Geometry: final body of the model. Coordinates: model frame, mm. Face numbers are marked on the shaded views. A direction names the side the tool comes from. Give positions to 0.01 mm unless a question says otherwise; leave off trailing zeros. Order: outer loops, then holes, each group sorted by start corner. A loop starts at its lowest first (then second) coordinate and runs counter-clockwise, first axis right, second up. Notation, with made-up numbers: (20.5, 54.25) - (66.5, 54.25) arc R9 ccw to (66.5, 61.25) - close; hole circle Ø3 at (-17, 38.25). An arc over 180 degrees is marked (long way). Write item = value, one per line. Start each with the question number.
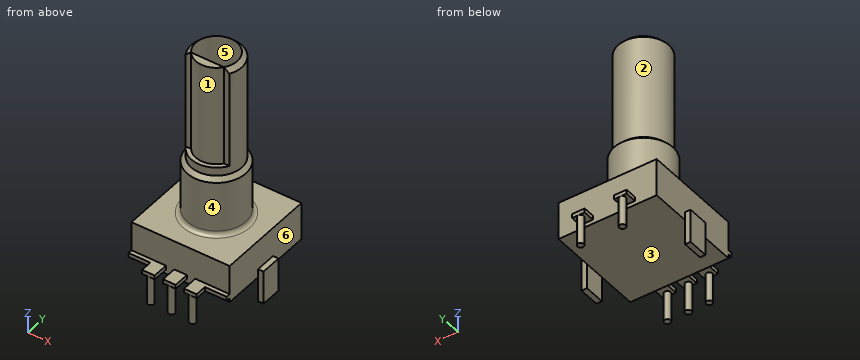
Autodesk Fusion 360 part; units mm, degrees
sketch "Skizze1" plane through (0, 0, 0) normal (0, 0, 1) x (1, 0, 0)
  line L0 (0, 0) -> (-11.7, 0)
  line L1 (-11.7, 0) -> (-11.7, 12)
  line L2 (-11.7, 12) -> (0, 12)
  line L3 (0, 12) -> (0, 0)
  dimension "d1" = 11.7
  dimension "d2" = 12
extrude "Extrusion1" add sketch "Skizze1" along normal blind 4.5
ref_plane "Arbeitsebene1" through (0, 0, 0.5) normal (0, 0, 1) x (1, 0, 0)
sketch "Skizze2" plane through (0, 0, 0.5) normal (0, 0, 1) x (1, 0, 0)
  line L0 (0, 12) -> (-11.7, 12)
  line L1 (-11.7, 12) -> (-11.7, 0)
  line L2 (-11.7, 0) -> (0, 0)
  line L3 (0, 0) -> (0, 12)
  line L4 (-8.35, 12) -> (-8.35, 19) construction
  line L5 (-3.35, 12) -> (-3.35, 19) construction
  line L6 (-8.35, 0) -> (-8.35, -5) construction
  line L7 (-5.85, 0) -> (-5.85, -5) construction
  line L8 (-3.35, 0) -> (-3.35, -5) construction
  line L9 (-7.6, 12) -> (-9.1, 12)
  line L10 (-9.1, 12) -> (-9.1, 13.375)
  line L11 (-9.1, 13.375) -> (-7.6, 13.375)
  line L12 (-7.6, 13.375) -> (-7.6, 12)
  line L13 (-2.6, 12) -> (-4.1, 12)
  line L14 (-4.1, 12) -> (-4.1, 13.375)
  line L15 (-4.1, 13.375) -> (-2.6, 13.375)
  line L16 (-2.6, 13.375) -> (-2.6, 12)
  line L17 (-2.6, 0) -> (-4.1, 0)
  line L18 (-4.1, 0) -> (-4.1, -1.875)
  line L19 (-4.1, -1.875) -> (-2.6, -1.875)
  line L20 (-2.6, -1.875) -> (-2.6, 0)
  line L21 (-6.6, 0) -> (-5.1, 0)
  line L22 (-5.1, 0) -> (-5.1, -1.875)
  line L23 (-5.1, -1.875) -> (-6.6, -1.875)
  line L24 (-6.6, -1.875) -> (-6.6, 0)
  line L25 (-9.1, 0) -> (-7.6, 0)
  line L26 (-7.6, 0) -> (-7.6, -1.875)
  line L27 (-7.6, -1.875) -> (-9.1, -1.875)
  line L28 (-9.1, -1.875) -> (-9.1, 0)
  line L29 (-9.1, 0) -> (-11.7, 0)
  line L30 (-11.7, 0) -> (-11.7, -0.5)
  line L31 (-11.7, -0.5) -> (-9.1, -0.5)
  line L32 (-9.1, -0.5) -> (-9.1, 0)
  line L33 (-2.6, 0) -> (0, 0)
  line L34 (0, 0) -> (0, -0.5)
  line L35 (0, -0.5) -> (-2.6, -0.5)
  line L36 (-2.6, -0.5) -> (-2.6, 0)
  circle A0 centre (-8.35, 13) radius 0.375
  circle A1 centre (-3.35, 13) radius 0.375
  circle A2 centre (-8.35, -1.5) radius 0.375
  circle A3 centre (-5.85, -1.5) radius 0.375
  circle A4 centre (-3.35, -1.5) radius 0.375
  line L37 (-11.7, 6) -> (0, 6) construction
  line L38 (-11.7, 7.25) -> (-12.35, 7.25)
  line L39 (-12.35, 7.25) -> (-12.35, 4.75)
  line L40 (-12.35, 4.75) -> (-11.7, 4.75)
  line L41 (-11.7, 4.75) -> (-11.7, 7.25)
  line L42 (0, 7.25) -> (0.65, 7.25)
  line L43 (0.65, 7.25) -> (0.65, 4.75)
  line L44 (0.65, 4.75) -> (0, 4.75)
  line L45 (0, 4.75) -> (0, 7.25)
  line L46 (-11.6, 7.25) -> (-11.6, 4.75)
  line L47 (-0.1, 7.25) -> (-0.1, 4.75)
  dimension "d7" = 5
  dimension "d8" = 5
  dimension "d9" = 1.5
  dimension "d11" = 0.5
  dimension "d12" = 0.75
  dimension "d13" = 0.75
  dimension "d14" = 0.75
  dimension "d15" = 0.75
  dimension "d16" = 0.75
  dimension "d17" = 7
  dimension "d18" = 7
  dimension "d19" = 7.5
  dimension "d20" = 7.5
  dimension "d21" = 7.5
  dimension "d26" = 0.75
  dimension "d27" = 0.75
  dimension "d28" = 13
  dimension "d46" = 2.5
extrude "Extrusion2" add sketch "Skizze2" along normal blind 0.5 contours A1 | L0 L13 L14 L15 L16 | L3 L42 L43 L44 L45 | A0 | L0 L9 L10 L11 L12 | L2 L20 L33 L34 L35 L36 | A4 | L2 L17 L18 L19 L20 L36 | L1 L38 L39 L40 L41 | A3 | L2 L21 L22 L23 L24 | L2 L28 L29 L30 L31 L32 | A2 | L2 L25 L26 L27 L28 L32
extrude "Extrusion3" add sketch "Skizze2" against normal blind 3.5 contours A1 | L3 L42 L43 L44 L45 | A0 | A4 | L1 L38 L39 L40 L41 | A3 | A2
ref_plane "Arbeitsebene2" through (0, 6, 0) normal (0, 1, 0) x (0, 0, 1)
sketch "Skizze3" plane through (0, 6, 0) normal (0, 1, 0) x (1, 0, 0)
  line L0 (-4.1, -1) -> (0, -1)
  line L1 (0, -1) -> (0, -4.5)
  line L2 (0, -4.5) -> (-11.7, -4.5)
  line L3 (-11.7, -4.5) -> (-11.7, -1)
  line L4 (-11.7, -1) -> (-7.6, -1)
  line L5 (-7.6, -1) -> (-7.6, -0.5)
  line L6 (-7.6, -0.5) -> (-11.7, -0.5)
  line L7 (-11.7, -0.5) -> (-11.7, 0)
  line L8 (-11.7, 0) -> (0, 0)
  line L9 (0, 0) -> (0, -0.5)
  line L10 (0, -0.5) -> (-4.1, -0.5)
  line L11 (-4.1, -0.5) -> (-4.1, -1)
  line L12 (-5.1, -1) -> (-5.1, -0.5)
  line L13 (-5.1, -0.5) -> (-6.6, -0.5)
  line L14 (-6.6, -0.5) -> (-6.6, -1)
  line L15 (-6.6, -1) -> (-5.1, -1)
  line L16 (-5.85, -4.5) -> (-5.85, -18.5)
  line L17 (-5.85, -4.5) -> (-1.85, -4.5)
  line L18 (-2.35, -5) -> (-2.35, -11)
  arc A0 (-1.85, -4.5) -> (-2.35, -5) centre (-1.85, -5) ccw
  line L19 (-2.35, -11) -> (-2.85, -11.5)
  line L20 (-2.85, -11.5) -> (-2.85, -23.9697)
  line L21 (-2.85, -23.9697) -> (-3.3803, -24.5)
  line L22 (-3.3803, -24.5) -> (-5.85, -24.5)
  line L23 (-5.85, -24.5) -> (-5.85, -4.5)
  dimension "d31" = 1
  dimension "d32" = 7
  dimension "d33" = 6
  dimension "d34" = 135
  dimension "d35" = 135
  dimension "d36" = 7
  dimension "d40" = 0.75
  dimension "d41" = 20
revolve "Drehen1" add sketch "Skizze3" angle 360 about axis through (-5.85, 6, 4.5) along (0, 0, 1) contours L2 L16 L17 L18 A0 L19 L20 L21 L22 L23
sketch "Skizze4" plane through (0, 0, 24.5) normal (0, 0, 1) x (-1, 0, 0)
  circle A0 centre (5.85, -6) radius 2.4697
  circle A1 centre (5.85, -6) radius 3
  line L0 (8.4481, -4.5) -> (3.2519, -4.5)
  arc A2 (8.4481, -4.5) -> (3.2519, -4.5) centre (5.85, -6) ccw
  line L1 (5.85, -4.5) -> (5.85, -9) construction
  dimension "d43" = 4.5
extrude "Extrusion4" cut sketch "Skizze4" against normal blind 12 contours A0 L0 | A0 A1 L0 A2 picked at (5.4755, -5.7331)
equation "d13 = d12"
equation "d14 = d12"
equation "d15 = d12"
equation "d16 = d12"
Q1. Section D-D, the plane y = 11. Return the cut outline in (x, z).
Q2. Material intervals for line 1 along Y through (x, z) = (-5.85, 20.5); line 2 along X through (y, z) = (6, 18.5); line 3 along Y through (x, z) = (-4, 3.75), sorted ascending. Write a range as from..to.
Q3. Section A-A, the plane y = -1.5. Return the cut outline in (x, z) (3 decimals).
Q4. Contact query for flat-ended pins moving along their axis: pin 1 (4.5 mm diameter, centred on x = -5.5, z = 19, fed in from +Y); pin 2 (4 mm diameter, centred on x = -10, y = 2.5, fed in from +Z); pin 3 (8 mm diameter, centred on y = 5, z = 9.5, fed in from +X). Output: stop coordinate, or through.
Q5. Section B-B, the plane y = 13. Return the cut outline in (x, z) (3 decimals).
Q6. Pull-direction query (Y, two-part tool) for the marked faces 4, 5 and 6; classes: +Y half, -Y half, draft (parallel to the pull), parting line (faces both ways), or undercut.
Q7. Set-up query: the marked faces 1, 2 and 3. Return all of +Z, -Z, +X, -X, +Y, -Y with unobstructed straight access to the full face (end or side cutting, diameter ignored); none if empty.
The answers:
q1.outline = (-11.7, 0) - (0, 0) - (0, 4.5) - (-11.7, 4.5) - close
q2.line_1 = 3.53..4.5, 8.47..9
q2.line_2 = -8.85..-8.32, -3.38..-2.85
q2.line_3 = 0..12
q3.outline = (-9.1, 0.5) - (-8.725, 0.5) - (-8.725, -3) - (-7.975, -3) - (-7.975, 0.5) - (-7.6, 0.5) - (-7.6, 1) - (-9.1, 1) - close; (-6.6, 0.5) - (-6.225, 0.5) - (-6.225, -3) - (-5.475, -3) - (-5.475, 0.5) - (-5.1, 0.5) - (-5.1, 1) - (-6.6, 1) - close; (-4.1, 0.5) - (-3.725, 0.5) - (-3.725, -3) - (-2.975, -3) - (-2.975, 0.5) - (-2.6, 0.5) - (-2.6, 1) - (-4.1, 1) - close
q4.pin_1 = 9
q4.pin_2 = 11.07
q4.pin_3 = -2.35
q5.outline = (-9.1, 0.5) - (-8.725, 0.5) - (-8.725, -3) - (-7.975, -3) - (-7.975, 0.5) - (-7.6, 0.5) - (-7.6, 1) - (-9.1, 1) - close; (-4.1, 0.5) - (-3.725, 0.5) - (-3.725, -3) - (-2.975, -3) - (-2.975, 0.5) - (-2.6, 0.5) - (-2.6, 1) - (-4.1, 1) - close
q6.face_4 = parting line
q6.face_5 = undercut
q6.face_6 = draft
q7.face_1 = +Z, -Y
q7.face_2 = +Z
q7.face_3 = -Z
